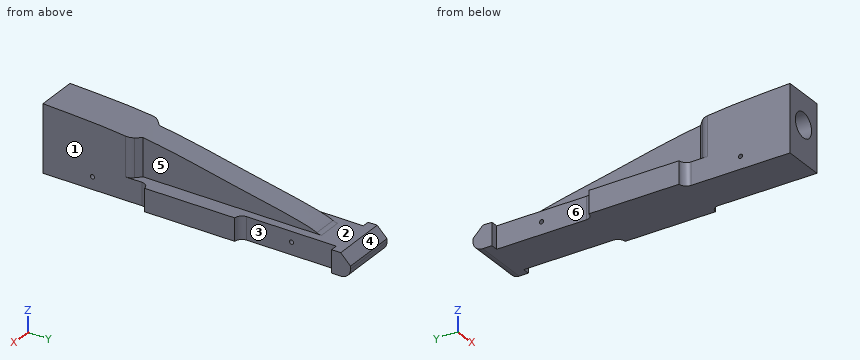
from build123d import *

# Parameters (mm, degrees)
F1_DEPTH  = 21.43125
F2_R      = 9.525
F3_DEPTH  = 50.8
F5_W      = 42.8625
F5_H      = 62.5831912994
F7_DEPTH  = 117.856
F8_W      = 5.55625
F8_H      = 69.85
F9_DEPTH  = 25.4
F10_DEPTH = 78.232
F12_DEPTH = 65.786
F14_DEPTH = 70.104
F16_DEPTH = 6.604
F17_SIZE  = 7.62
F18_R     = 7.62
F19_SIZE  = 6.35
F20_R     = 7.62
F21_R     = 1.5875
F22_DEPTH = 32.258
F23_R     = 1.5875
F24_DEPTH = 36.068


with BuildPart() as f1:
    # F0 (on Right) → F1 (new body, symmetric)
    with BuildSketch(Plane.YZ):
        Polygon((-152.4, 69.85), (-152.4, 0), (152.4, 0), (152.4, 19.05), align=None)
    extrude(amount=F1_DEPTH, both=True)

    # F2 (on face) → F3 (cut)
    with BuildSketch(Plane.XZ.offset(152.4)):
        with Locations((0, 34.925)):
            Circle(F2_R)
    extrude(amount=-F3_DEPTH, mode=Mode.SUBTRACT)

    # F5 (on face) → F7 (cut)
    with BuildSketch(Plane(origin=(0, 0, 0), x_dir=(1, 0, 0), z_dir=(0, 0, -1))):
        with BuildLine():
            Line((-15.875, 75.6509676576), (-15.875, 95.25))
            Line((-15.875, 95.25), (-15.875, 152.4))
            Line((-15.875, 152.4), (-21.43125, 152.1471400823))
            Line((-21.43125, 152.1471400823), (-21.43125, 70.0947176576))
            ThreePointArc((-21.43125, 70.0947176576), (-17.502387947, 71.7221056046), (-15.875, 75.6509676576))
        make_face()
        with BuildLine():
            Line((15.86865, -75.1233920455), (21.43125, -75.1233920455))
            Line((21.43125, -75.1233920455), (21.43125, -5.5626))
            Line((21.43125, -5.5626), (21.43125, 0))
            ThreePointArc((21.43125, 0), (17.497897819, -1.629247819), (15.86865, -5.5626))
            Line((15.86865, -5.5626), (15.86865, -43.3772839606))
            Line((15.86865, -43.3772839606), (15.86865, -75.1233920455))
        make_face()
        with Locations((0, -121.1084043503)):
            Rectangle(F5_W, F5_H)
        with BuildLine():
            ThreePointArc((-15.86865, -5.5626), (-17.497897819, -1.629247819), (-21.43125, 0))
            Line((-21.43125, 0), (-21.43125, -75.1233920455))
            Line((-21.43125, -75.1233920455), (-15.86865, -75.1233920455))
            Line((-15.86865, -75.1233920455), (-15.86865, -43.3772839606))
            Line((-15.86865, -43.3772839606), (-15.86865, -5.5626))
        make_face()
        with BuildLine():
            Line((21.43125, 152.4), (15.875, 152.4))
            Line((15.875, 152.4), (15.875, 95.25))
            Line((15.875, 95.25), (15.875, 75.6509676576))
            ThreePointArc((15.875, 75.6509676576), (17.502387947, 71.7221056046), (21.43125, 70.0947176576))
            Line((21.43125, 70.0947176576), (21.43125, 152.4))
        make_face()
    extrude(amount=-F7_DEPTH, mode=Mode.SUBTRACT)

    # F8 (on face) → F9 (cut)
    with BuildSketch(Plane.XZ.offset(152.4)):
        with Locations((-18.653125, 34.925)):
            Rectangle(F8_W, F8_H)
    extrude(amount=-F9_DEPTH, mode=Mode.SUBTRACT)

    # F4 (on face) → F10 (cut)
    with BuildSketch(Plane.YZ.offset(21.43125)):
        with BuildLine():
            Line((-166.5327996016, 95.561735332), (-152.4, 58.5300065577))
            add(Edge.make_bspline(
                [(-152.4, 58.5300065577), (-131.9690523131, 57.5975989918), (-92.9028985073, 56.6319201488), (-39.12835213, 46.6520301008), (-5.7136492039, 39.0230650087), (52.8600042471, 28.1535812859), (57.15, 24.1312850267)],
                knots=[0, 0, 0, 0, 0.2679549114, 0.514366781, 0.7364046279, 1, 1, 1, 1], degree=3))
            Line((57.15, 24.1312850267), (166.3713157177, 24.1312850267))
            Line((166.3713157177, 24.1312850267), (-166.5327996016, 95.561735332))
        make_face()
    extrude(amount=-F10_DEPTH, mode=Mode.SUBTRACT)

    # F11 (on face) → F12 (cut)
    with BuildSketch(Plane.XY.offset(24.1312850267)):
        Polygon((26.5305805951, 75.1233920455), (15.86865, 75.1233920455), (9.51865, 75.1233920455), (9.51865, -78.8636729121), (26.5305805951, -78.8636729121), align=None)
    extrude(amount=F12_DEPTH, mode=Mode.SUBTRACT)

    # F13 (on face) → F14 (cut)
    with BuildSketch(Plane.XY.offset(24.1312850267)):
        Polygon((-9.51865, 57.15), (-15.86865, 57.15), (-28.360279277, 57.15), (-37.0513312519, -78.8636729121), (-9.51865, -78.8636729121), align=None)
    extrude(amount=F14_DEPTH, mode=Mode.SUBTRACT)

    # F6 (on face) → F16 (cut)
    with BuildSketch(Plane(origin=(0, 0, 0), x_dir=(1, 0, 0), z_dir=(0, 0, -1))):
        with BuildLine():
            Line((15.875, 75.6509676576), (15.875, 95.25))
            Line((15.875, 95.25), (15.875, 152.4))
            Line((15.875, 152.4), (-15.875, 152.4))
            Line((-15.875, 152.4), (-15.875, 95.25))
            Line((-15.875, 95.25), (-15.875, 75.6509676576))
            ThreePointArc((-15.875, 75.6509676576), (-17.502387947, 71.7221056046), (-21.43125, 70.0947176576))
            Line((-21.43125, 70.0947176576), (-21.43125, 0))
            ThreePointArc((-21.43125, 0), (-17.497897819, -1.629247819), (-15.86865, -5.5626))
            Line((-15.86865, -5.5626), (-15.86865, -43.3772839606))
            Line((-15.86865, -43.3772839606), (-15.86865, -75.1233920455))
            Line((-15.86865, -75.1233920455), (-21.43125, -75.1233920455))
            Line((-21.43125, -75.1233920455), (-21.43125, -89.8168087006))
            Line((-21.43125, -89.8168087006), (21.43125, -89.8168087006))
            Line((21.43125, -89.8168087006), (21.43125, -75.1233920455))
            Line((21.43125, -75.1233920455), (15.86865, -75.1233920455))
            Line((15.86865, -75.1233920455), (15.86865, -43.3772839606))
            Line((15.86865, -43.3772839606), (15.86865, -5.5626))
            ThreePointArc((15.86865, -5.5626), (17.497897819, -1.629247819), (21.43125, 0))
            Line((21.43125, 0), (21.43125, 70.0947176576))
            ThreePointArc((21.43125, 70.0947176576), (17.502387947, 71.7221056046), (15.875, 75.6509676576))
        make_face()
    extrude(amount=-F16_DEPTH, mode=Mode.SUBTRACT)

    # F17
    f17_edges = [f1.edges().sort_by_distance(p)[0] for p in [
        (0, 89.816809, 24.131285),
    ]]
    chamfer(f17_edges, length=F17_SIZE)

    # F18
    f18_edges = [f1.edges().sort_by_distance(p)[0] for p in [
        (0, 89.816809, 6.604),
        (0, 57.15, 24.131285),
    ]]
    fillet(f18_edges, radius=F18_R)

    # F19
    f19_edges = [f1.edges().sort_by_distance(p)[0] for p in [
        (-15.875, -78.863673, 38.753924),
        (15.875, -78.863673, 38.753924),
    ]]
    chamfer(f19_edges, length=F19_SIZE)

    # F20
    f20_edges = [f1.edges().sort_by_distance(p)[0] for p in [
        (-15.875, -85.213673, 39.172756),
        (15.875, -85.213673, 39.172756),
    ]]
    fillet(f20_edges, radius=F20_R)

    # F21 (on face) → F22 (cut)
    with BuildSketch(Plane.YZ.offset(15.875)):
        with Locations((-114.0254838288, 16.129)):
            Circle(F21_R)
    extrude(amount=-F22_DEPTH, mode=Mode.SUBTRACT)

    # F23 (on face) → F24 (cut)
    with BuildSketch(Plane.YZ.offset(15.86865)):
        with Locations((40.3429960227, 16.129)):
            Circle(F23_R)
    extrude(amount=-F24_DEPTH, mode=Mode.SUBTRACT)


solid = f1.part
Here's how the part is built. I have some questions about the finished solid (model axes, mm). Face numbers are marked on the shaded views. A direction names the side the tool comes from. Give positions to 0.01 mm unless a question says otherwise; leave off trailing zeros. Write each loop counter-clockwise with the first axis right and the second up, starting at its lowest first coordinate (ties: lowest second). Pieces come first, ordered by that corner, then holes. Notation, with made-up numbers: (-7, 45) -> (-2, 45) arc R18 ccw to (-2, 78) -> close; hole circle Ø2 at (19.25, 53.25). An arc over 180 degrees is marked (long way). Use one line per item in the form item = value. Start each with the question number.
1. Imagine slicing it at B-B on z = 12. List the corners of the cut face in (x, y) for me (1 decimal).
2. Thinking about a two-plate mould opening in Y: for the marked faces 4, 5 and 6, which applies, +Y half, -Y half, draft (parallel to the pull), parting line (faces both ways), or undercut?
3. Imagine slicing it at A-A on x = -18. List the corners of the cut face in (y, z) for me, plus the area to 3 significant figures.
4. Will these pins go through, and if not, where does the flat tip stop? pin 1 Ø2 at (x, y) = (9, -96) entering from +Z; pin 2 Ø9 at (y, z) = (47, 12.5) entering from -X; pin 3 Ø10 at (x, y) = (-5, -94) entering from +Z; pin 4 Ø1.9 at (y, z) = (40.34, 16.13) entering from -X.
5. On a 3-axis mill with a long thin cutter (end or side, diameter ignored), from which of +Z, -Z, +X, -X, +Y, -Y can I reach the whole of each face in a straight line? I mean the marked faces 1, 2 and 3. Say none if no direction works.
6. Imagine slicing it at D-D on y = 63. List the corners of the cut face in (x, z) for me, plus the area to 3 significant figures.
7. Imagine slicing it at C-C on x = 2. State how many separate pieces and enclosed holes the cut face has, plus the area to 3 significant figures.
8. If I drill on L1, parallel to Z at x = 15, y = -5; L2, parallel to X at y = -4.5, z = 29.5; L3, parallel to Y at x = 14, z = 15, over which ranges is the centre line in solid material (lowest first)?
Entries:
q1.outline = (-21.4, -70.1) arc R5.6 cw to (-15.9, -75.7) -> (-15.9, -152.4) -> (15.9, -152.4) -> (15.9, -75.7) arc R5.6 cw to (21.4, -70.1) -> (21.4, 0) arc R5.6 cw to (15.9, 5.6) -> (15.9, 75.1) -> (21.4, 75.1) -> (21.4, 89.5) -> (-21.4, 89.5) -> (-21.4, 75.1) -> (-15.9, 75.1) -> (-15.9, 5.6) arc R5.6 cw to (-21.4, 0) -> close
q2.face_4 = +Y half
q2.face_5 = draft
q2.face_6 = undercut
q3.outline = (-71.28, 6.6) -> (1.18, 6.6) -> (1.18, 24.13) -> (-71.28, 24.13) -> close; (75.12, 6.6) -> (82.2, 6.6) arc R7.62 ccw to (89.82, 14.22) -> (89.82, 16.51) -> (82.2, 24.13) -> (75.12, 24.13) -> close
q3.area = 1,490 mm²
q4.pin_1 = 55.49
q4.pin_2 = -15.87
q4.pin_3 = 55.67
q4.pin_4 = through
q5.face_1 = +Z, -Z, +X, -Y
q5.face_2 = +Z, +Y
q5.face_3 = +Z, -Z, +X
q6.outline = (-15.87, 6.6) -> (15.87, 6.6) -> (15.87, 24.13) -> (-15.87, 24.13) -> close
q6.area = 556 mm²
q7.separate_pieces = 1
q7.enclosed_holes = 2
q7.area = 7,830 mm²
q8.L1 = 6.6 to 24.13
q8.L2 = -9.52 to 9.52
q8.L3 = -152.4 to -115.14, -112.91 to 39.23, 41.46 to 89.82
